```python
from build123d import *

# Parameters (mm, degrees)
F0_W     = 79.84292
F0_H     = 57.80068
F1_DEPTH = 25.4
F2_R     = 4.412951
F3_DEPTH = 25.4
F4_T     = -2.54


with BuildPart() as f1:
    # F0 (on Front) → F1 (new body)
    with BuildSketch(Plane.XZ):
        with Locations((-50.115223, 20.620596)):
            Rectangle(F0_W, F0_H)
    extrude(amount=F1_DEPTH)

    # F2 (on face) → F3 (cut)
    with BuildSketch(Plane.XZ.offset(25.4)):
        with Locations((-79.845399, 7.352189)):
            Circle(F2_R)
    extrude(amount=-F3_DEPTH, mode=Mode.SUBTRACT)

    # F4
    f4_openings = [f1.faces().sort_by_distance(p)[0] for p in [
        (-49.715801, 0, 20.798856),
    ]]
    offset(amount=F4_T, openings=f4_openings)


solid = f1.part
```
Input: part model. Units: mm. Frame: model coordinates. A direction names the side the tool comes from. Coordinates: 2 decimals unless noted, no trailing zeros. Loops run counter-clockwise (first coordinate to the right, second up) from the corner with the lowest first, then second, coordinate; pieces in that order, holes last. Notation, with made-up numbers: (15, 61) - (23, 61) arc R31 ccw to (23, 91) - close; hole circle Ø2 at (30, 23). An arc over 180 degrees is marked (long way). Answer in a Markdown table with one row per item.
(1) Cut plane B-B on x = -43. Output: boundary loops of the cut face in (y, z), plus the area to 3 significant figures.
Model answer:
| item | result |
|---|---|
| outline | (-25.4, -8.28) - (0, -8.28) - (0, -5.74) - (-22.86, -5.74) - (-22.86, 46.98) - (0, 46.98) - (0, 49.52) - (-25.4, 49.52) - close |
| area | 263 mm² |
(2) Cut plane D-D on x = -80. Output: boundary loops of the cut face in (y, z).
Model answer:
| item | result |
|---|---|
| outline | (-25.4, -8.28) - (0, -8.28) - (0, -5.74) - (-22.86, -5.74) - (-22.86, 0.4) - (0, 0.4) - (0, 2.94) - (-25.4, 2.94) - close; (-25.4, 11.76) - (0, 11.76) - (0, 14.3) - (-22.86, 14.3) - (-22.86, 46.98) - (0, 46.98) - (0, 49.52) - (-25.4, 49.52) - close |
(3) Cut plane C-C on z = 23. Output: boundary loops of the cut face in (x, y), plus the area to 3 significant figures.
Model answer:
| item | result |
|---|---|
| outline | (-90.04, -25.4) - (-10.19, -25.4) - (-10.19, 0) - (-12.73, 0) - (-12.73, -22.86) - (-87.5, -22.86) - (-87.5, 0) - (-90.04, 0) - close |
| area | 319 mm² |
(4) Material intervals for L1, parallel to X at y = -13.5, z = 7; L2, parallel to X at y = -16.25, z = -0.5; L3, parallel to Z at x = -54.5, y = -3, sorted ascending. Write a range as from..to.
Model answer:
| item | result |
|---|---|
| L1 | x = -90.04..-87.5, -86.79..-84.24, -75.45..-72.9, -12.73..-10.19 |
| L2 | x = -90.04..-87.5, -12.73..-10.19 |
| L3 | z = -8.28..-5.74, 46.98..49.52 |
(5) Cut plane A-A on y = -18.25. Output: boundary loops of the cut face in (x, z).
Model answer:
| item | result |
|---|---|
| outline | (-90.04, -8.28) - (-10.19, -8.28) - (-10.19, 49.52) - (-90.04, 49.52) - close; circle Ø13.91 at (-79.85, 7.35); hole (-87.5, -5.74) - (-12.73, -5.74) - (-12.73, 46.98) - (-87.5, 46.98) - close; hole circle Ø8.83 at (-79.85, 7.35) |
(6) Pin query (flat end, axial travel): P1, Ø8, axis at x = -25, z = 41, coming from the +Y side. Return the tip coordinate at first contact, or that it passes through.
Model answer:
| item | result |
|---|---|
| P1 | stops at y = -22.86 |
(7) Mould query, pull axis X, two halves, no side actions, for faces 1 (the face through (-51, -13, -8.28)), 2 (the face through (-90.037, -13, 20)), 3 (the face through (-51, -11, 46.981)). Classes: pulls with the +X half, pulls with the -X half, needs draft (parallel to the pull), parting line crosses it, or undercut.
Model answer:
| item | result |
|---|---|
| face 1 | needs draft |
| face 2 | pulls with the -X half |
| face 3 | undercut |
(8) Set-up query: faces 4 (the face through (-12.734, -11, 20)), 5 (the face through (-75, 0, 7)). Return all of +Z, -Z, +X, -X, +Y, -Y with unobstructed straight access to the full face (end or side cutting, diameter ignored); none if empty.
Model answer:
| item | result |
|---|---|
| face 4 | +Y |
| face 5 | +Z, -Z, +X, -X, +Y |
